Build history of the part. All positions in model axes, mm. A direction names the side the tool comes from. Round coordinates to 2 decimals unless told otherwise and drop trailing zeros. Write each loop counter-clockwise with the first axis right and the second up, starting at its lowest first coordinate (ties: lowest second). Pieces come first, ordered by that corner, then holes. Notation, with made-up numbers: (26.5, 44) - (68.5, 44) arc R30 cw to (68.5, 80) - close; hole circle Ø4 at (36, 73). An arc over 180 degrees is marked (long way). Answer as a JSON object with one key per item and string values. Group by question number.
Item 1: Which spindle directions (+Z, -Z, +X, -X, +Y, -Y) get a long thin tool onto all of the face, cutting with end or side? Do faces 4 (the cylindrical face through (80.406, -16.369, -0.686)), 5 (the flat face through (-103.5, -6, 53)), 6 (the cylindrical face through (106.975, -5.07, 79.019)). Say none if no direction does.
Item 2: Two-plate mould, pull along Z, no slides. Class faces 1 (the cylindrical face through (-1.155, -15.719, 86.594)), 2 (the flat face through (-1, -6, -78)), 3 (the flat face through (-117.5, -5, -1)): +Z half, -Z half, draft (parallel to the pull), parting line (faces both ways), or undercut.
Item 3: Slice it at B-B, the plane z = 2. List the corners of the cut face in (x, y).
Item 4: Slice it at C-C, the plane y = -5.75. List the corners of the cut face in (x, z), then the cut area to 3 significant figures.
Item 5: Slice it at A-A, the plane x = 43. List the corners of the cut face in (y, z), then the cut area to 3 significant figures.
Item 6: Probe line 1 (Z direction, x = 4.5, y = -8.5); line 2 (X direction, y = -10, z = 10); line 3 (Y direction, x = -25, z = -65). List the from-to ranges inside material, lowest first. Write a range as from..to.
Item 7: Flat gauge pins, fed straight in: pin 1 (8 mm diameter, centred on x = -89.5, y = -14.5, fed in from -Z); pin 2 (6 mm diameter, centred on y = -5.5, z = -64, fed in from +X); pin 3 (8 mm diameter, centred on x = 44.5, z = -66, fed in from +Y). Where does each tip first touch, or does it go through?
from build123d import *

# Parameters (mm, degrees)
F0_W         = 235
F0_H         = 178
F0_W_2       = 207
F0_H_2       = 156
F0_W_3       = 155
F0_H_3       = 106
F1_DEPTH     = 18
F2_DEPTH     = 12
F3_R         = 35
F4_R         = 4
F5_T1_DEPTH  = 98
F5_T3_DEPTH  = 147
F5_T5_DEPTH  = 165
F5_T7_DEPTH  = 108
F5_T10_ANGLE = 90
F5_T12_ANGLE = 90
F5_T14_ANGLE = 90
F5_T16_ANGLE = 90
F5_T18_ANGLE = 90
F5_T20_ANGLE = 90
F5_T22_ANGLE = 90
F5_T24_ANGLE = 90
F6_SIZE      = 3
F7_R         = 1.5
F8_DEPTH     = 16


# Not quite as in the source:
# - a fillet or chamfer that OpenCascade refuses, or shapes differently, is made with other operations: its cross-section is extruded or revolved along the edge and cut away or added


with BuildPart() as f1:
    # F0 (on Front) → F1 (new body)
    with BuildSketch(Plane.XZ):
        Rectangle(F0_W, F0_H)
        Rectangle(F0_W_2, F0_H_2, mode=Mode.SUBTRACT)
        Rectangle(F0_W_2, F0_H_2)
        Rectangle(F0_W_3, F0_H_3, mode=Mode.SUBTRACT)
    extrude(amount=F1_DEPTH)

    # F0 (on Front) → F2 (cut)
    with BuildSketch(Plane.XZ):
        Rectangle(F0_W_2, F0_H_2)
        Rectangle(F0_W_3, F0_H_3, mode=Mode.SUBTRACT)
    extrude(amount=F2_DEPTH, mode=Mode.SUBTRACT)

    # F3
    f3_edges = [f1.edges().sort_by_distance(p)[0] for p in [
        (117.5, -9, 89),
        (-117.5, -9, 89),
        (117.5, -9, -89),
        (-117.5, -9, -89),
    ]]
    fillet(f3_edges, radius=F3_R)

    # F4
    f4_edges = [f1.edges().sort_by_distance(p)[0] for p in [
        (-77.5, -15, 53),
        (77.5, -15, 53),
        (77.5, -15, -53),
        (-77.5, -15, -53),
    ]]
    fillet(f4_edges, radius=F4_R)

    # F5: fillet of radius 8 on 16 edges, made by hand

    # F5_s2 → F5_t1 (cut)
    with BuildSketch(Plane.XY.offset(-49)):
        with BuildLine():
            ThreePointArc((-85.2459666924, -18), (-80.3469872068, -16.3245553203), (-77.5, -12))
            Line((-77.5, -12), (-77.5, -18))
            Line((-77.5, -18), (-85.2459666924, -18))
        make_face()
        with BuildLine():
            ThreePointArc((85.2459666924, -18), (80.3469872068, -16.3245553203), (77.5, -12))
            Line((77.5, -12), (77.5, -18))
            Line((77.5, -18), (85.2459666924, -18))
        make_face()
    extrude(amount=F5_T1_DEPTH, mode=Mode.SUBTRACT)

    # F5_s4 → F5_t3 (cut)
    with BuildSketch(Plane.YZ.offset(-73.5)):
        with BuildLine():
            ThreePointArc((-18, -60.7459666924), (-16.3245553203, -55.8469872068), (-12, -53))
            Line((-12, -53), (-18, -53))
            Line((-18, -53), (-18, -60.7459666924))
        make_face()
        with BuildLine():
            ThreePointArc((-18, 60.7459666924), (-16.3245553203, 55.8469872068), (-12, 53))
            Line((-12, 53), (-18, 53))
            Line((-18, 53), (-18, 60.7459666924))
        make_face()
    extrude(amount=F5_T3_DEPTH, mode=Mode.SUBTRACT)

    # F5_s6 → F5_t5 (cut)
    with BuildSketch(Plane.YZ.offset(-82.5)):
        with BuildLine():
            ThreePointArc((-18, -81), (-15.6568542495, -86.6568542495), (-10, -89))
            Line((-10, -89), (-18, -89))
            Line((-18, -89), (-18, -81))
        make_face()
        with BuildLine():
            ThreePointArc((-18, 81), (-15.6568542495, 86.6568542495), (-10, 89))
            Line((-10, 89), (-18, 89))
            Line((-18, 89), (-18, 81))
        make_face()
    extrude(amount=F5_T5_DEPTH, mode=Mode.SUBTRACT)

    # F5_s8 → F5_t7 (cut)
    with BuildSketch(Plane.XY.offset(-54)):
        with BuildLine():
            ThreePointArc((-109.5, -18), (-115.1568542495, -15.6568542495), (-117.5, -10))
            Line((-117.5, -10), (-117.5, -18))
            Line((-117.5, -18), (-109.5, -18))
        make_face()
        with BuildLine():
            ThreePointArc((109.5, -18), (115.1568542495, -15.6568542495), (117.5, -10))
            Line((117.5, -10), (117.5, -18))
            Line((117.5, -18), (109.5, -18))
        make_face()
    extrude(amount=F5_T7_DEPTH, mode=Mode.SUBTRACT)

    # F5_s9 → F5_t10 (revolve, cut)
    with BuildSketch(Plane.XY.offset(-49)):
        with BuildLine():
            ThreePointArc((-85.2459666924, -18), (-80.3469872068, -16.3245553203), (-77.5, -12))
            Line((-77.5, -12), (-77.5, -18))
            Line((-77.5, -18), (-85.2459666924, -18))
        make_face()
    revolve(axis=Axis((-73.5, -18, -49), (0, -1, 0)), revolution_arc=F5_T10_ANGLE, mode=Mode.SUBTRACT)

    # F5_s11 → F5_t12 (revolve, cut)
    with BuildSketch(Plane.XY.offset(49)):
        with BuildLine():
            ThreePointArc((-85.2459666924, -18), (-80.3469872068, -16.3245553203), (-77.5, -12))
            Line((-77.5, -12), (-77.5, -18))
            Line((-77.5, -18), (-85.2459666924, -18))
        make_face()
    revolve(axis=Axis((-73.5, -18, 49), (0, 1, 0)), revolution_arc=F5_T12_ANGLE, mode=Mode.SUBTRACT)

    # F5_s13 → F5_t14 (revolve, cut)
    with BuildSketch(Plane.XY.offset(-49)):
        with BuildLine():
            ThreePointArc((85.2459666924, -18), (80.3469872068, -16.3245553203), (77.5, -12))
            Line((77.5, -12), (77.5, -18))
            Line((77.5, -18), (85.2459666924, -18))
        make_face()
    revolve(axis=Axis((73.5, -18, -49), (0, 1, 0)), revolution_arc=F5_T14_ANGLE, mode=Mode.SUBTRACT)

    # F5_s15 → F5_t16 (revolve, cut)
    with BuildSketch(Plane.YZ.offset(73.5)):
        with BuildLine():
            ThreePointArc((-18, 60.7459666924), (-16.3245553203, 55.8469872068), (-12, 53))
            Line((-12, 53), (-18, 53))
            Line((-18, 53), (-18, 60.7459666924))
        make_face()
    revolve(axis=Axis((73.5, -18, 49), (0, 1, 0)), revolution_arc=F5_T16_ANGLE, mode=Mode.SUBTRACT)

    # F5_s17 → F5_t18 (revolve, cut)
    with BuildSketch(Plane.YZ.offset(-82.5)):
        with BuildLine():
            ThreePointArc((-18, -81), (-15.6568542495, -86.6568542495), (-10, -89))
            Line((-10, -89), (-18, -89))
            Line((-18, -89), (-18, -81))
        make_face()
    revolve(axis=Axis((-82.5, -18, -54), (0, 1, 0)), revolution_arc=F5_T18_ANGLE, mode=Mode.SUBTRACT)

    # F5_s19 → F5_t20 (revolve, cut)
    with BuildSketch(Plane.YZ.offset(82.5)):
        with BuildLine():
            ThreePointArc((-18, -81), (-15.6568542495, -86.6568542495), (-10, -89))
            Line((-10, -89), (-18, -89))
            Line((-18, -89), (-18, -81))
        make_face()
    revolve(axis=Axis((82.5, -18, -54), (0, -1, 0)), revolution_arc=F5_T20_ANGLE, mode=Mode.SUBTRACT)

    # F5_s21 → F5_t22 (revolve, cut)
    with BuildSketch(Plane.XY.offset(54)):
        with BuildLine():
            ThreePointArc((-109.5, -18), (-115.1568542495, -15.6568542495), (-117.5, -10))
            Line((-117.5, -10), (-117.5, -18))
            Line((-117.5, -18), (-109.5, -18))
        make_face()
    revolve(axis=Axis((-82.5, -18, 54), (0, 1, 0)), revolution_arc=F5_T22_ANGLE, mode=Mode.SUBTRACT)

    # F5_s23 → F5_t24 (revolve, cut)
    with BuildSketch(Plane.XY.offset(54)):
        with BuildLine():
            ThreePointArc((109.5, -18), (115.1568542495, -15.6568542495), (117.5, -10))
            Line((117.5, -10), (117.5, -18))
            Line((117.5, -18), (109.5, -18))
        make_face()
    revolve(axis=Axis((82.5, -18, 54), (0, -1, 0)), revolution_arc=F5_T24_ANGLE, mode=Mode.SUBTRACT)

    # F6
    f6_edges = [f1.edges().sort_by_distance(p)[0] for p in [
        (-103.5, -6, -78),
        (103.5, -6, -78),
        (-103.5, -6, 78),
        (103.5, -6, 78),
    ]]
    chamfer(f6_edges, length=F6_SIZE)

    # F7 (on face) → F8 (join)
    with BuildSketch(Plane.XZ):
        with Locations((-103.5, -30)):
            Circle(F7_R)
        with Locations((-103.5, 30)):
            Circle(F7_R)
        with Locations((103.5, -30)):
            Circle(F7_R)
        with Locations((103.5, 30)):
            Circle(F7_R)
    extrude(amount=F8_DEPTH)


solid = f1.part
Geometry says:
{
 "1": {"face 4": "-Y", "face 5": "+Y", "face 6": "+Z, +X, +Y, -Y"},
 "2": {"face 1": "+Z half", "face 2": "undercut", "face 3": "draft"},
 "3": {"outline": "(-117.5, -10) arc R8 ccw to (-109.5, -18) - (-85.25, -18) arc R8 ccw to (-77.5, -12) - (-103.5, -12) - (-103.5, 0) - (-117.5, 0) - close; (77.5, -12) arc R8 ccw to (85.25, -18) - (109.5, -18) arc R8 ccw to (117.5, -10) - (117.5, 0) - (103.5, 0) - (103.5, -12) - close"},
 "4": {"outline": "(-117.5, -54) arc R35 ccw to (-82.5, -89) - (82.5, -89) arc R35 ccw to (117.5, -54) - (117.5, 54) arc R35 ccw to (82.5, 89) - (-82.5, 89) arc R35 ccw to (-117.5, 54) - close; hole (-103.5, -75) - (-100.5, -78) - (100.5, -78) - (103.5, -75) - (103.5, -31.5) arc R1.5 cw to (103.5, -28.5) - (103.5, 28.5) arc R1.5 cw to (103.5, 31.5) - (103.5, 75) - (100.5, 78) - (-100.5, 78) - (-103.5, 75) - (-103.5, 31.5) arc R1.5 cw to (-103.5, 28.5) - (-103.5, -28.5) arc R1.5 cw to (-103.5, -31.5) - close", "area": "8,520 mm^2"},
 "5": {"outline": "(-18, -81) arc R8 ccw to (-10, -89) - (0, -89) - (0, -78) - (-12, -78) - (-12, -53) arc R8 ccw to (-18, -60.75) - close; (-18, 60.75) arc R8 ccw to (-12, 53) - (-12, 78) - (0, 78) - (0, 89) - (-10, 89) arc R8 ccw to (-18, 81) - close", "area": "644 mm^2"},
 "6": {"line 1": "z = -89..-78, 78..89", "line 2": "x = -117.5..-103.5, 103.5..117.5", "line 3": "y = -18..-12"},
 "7": {"pin 1": "stops at z = -88.59", "pin 2": "stops at x = 116.79", "pin 3": "stops at y = -12"}
}
